Check sheet for the modelled part. Datum: model origin and axes. Units: mm. Round coordinates to 2 decimals unless told otherwise and drop trailing zeros. Write each loop counter-clockwise with the first axis right and the second up, starting at its lowest first coordinate (ties: lowest second). Pieces come first, ordered by that corner, then holes. Notation, with made-up numbers: M -8.5,39 L 8.5,39 A22 ccw 8.5,54 Z; hole C 14,82.25 d7. An arc over 180 degrees is marked long. Put each result on its own line as item: value.
```python
from build123d import *

# Parameters (mm, degrees)
F0_W = 40
F0_H = 7.5
F2_T = -1


with BuildPart() as f1:
    # F0 (on Top) → F1 (revolve)
    with BuildSketch(Plane.XY):
        with Locations((-23.359164299, 3.75)):
            Rectangle(F0_W, F0_H)
    revolve(axis=Axis((-23.359164299, 0, 0), (1, 0, 0)))

    # F2
    f2_openings = [f1.faces().sort_by_distance(p)[0] for p in [
        (-43.359164, 0, 0),
    ]]
    offset(amount=F2_T, openings=f2_openings)

    # F0 (on Top) → F3 (revolve)
    with BuildSketch(Plane.XY):
        with BuildLine():
            Line((-3.359164299, 10), (-3.359164299, 7.5))
            Line((-3.359164299, 7.5), (-3.359164299, 0))
            Line((-3.359164299, 0), (16.640835701, 0))
            add(Edge.make_bspline(
                [(13.8242446614, 5.8201136691), (15.4706541093, 3.8634896533), (16.522999446, 1.3952228585), (16.640835701, 0)],
                knots=[0.7411708943, 0.7411708943, 0.7411708943, 0.7411708943, 1, 1, 1, 1], degree=3))
            add(Edge.make_bspline(
                [(-3.359164299, 10), (-2.6756685908, 9.3742873677), (1.833779877, 8.8504755161), (9.6760817872, 9.8620826294), (13.1808157461, 6.5847767181), (13.8242446614, 5.8201136691)],
                knots=[0, 0, 0, 0, 0.2582901973, 0.6400185771, 0.7411708943, 0.7411708943, 0.7411708943, 0.7411708943], degree=3))
        make_face()
        with BuildLine():
            add(Edge.make_bspline(
                [(13.8242446614, 5.8201136691), (15.4706541093, 3.8634896533), (16.522999446, 1.3952228585), (16.640835701, 0)],
                knots=[0.7411708943, 0.7411708943, 0.7411708943, 0.7411708943, 1, 1, 1, 1], degree=3))
            Line((16.640835701, 0), (35.6210991124, 0))
            Line((35.6210991124, 0), (18.3005910367, 10))
            ThreePointArc((18.3005910367, 10), (17.4707133688, 10.4231546702), (16.640835701, 10))
            ThreePointArc((16.640835701, 10), (14.9843806263, 8.0772776447), (13.8242446614, 5.8201136691))
        make_face()
    revolve(axis=Axis((6.640835701, 0, 0), (1, 0, 0)))


solid = f1.part
```
1. Cross-section at B-B (x = 30). Enter the section's corners in (y, z), then the cut area to 3 significant figures.
Computed values:
outline: C 0,0 d6.49
area: 33.1 mm2
2. Cross-section at A-A (x = -34.5). Enter the section's corners in (y, z), then the cut area to 3 significant figures.
Computed values:
outline: C 0,0 d15; hole C 0,0 d13
area: 44.0 mm2
3. Release check for a two-part mould opening along Y. For faces 1 (the flat face through (-43.359, 6, 3)), 2 (the flat face through (-4.359, 0, 0)), 3 (the conical face through (28.764, -0.858, -3.865)) record: +Y half, -Y half, draft (parallel to the pull), parting line (faces both ways), or undercut.
Computed values:
face 1: draft
face 2: undercut
face 3: parting line
4. Scan lines: probe 1 along Z at (x, y) = (-22.5, 0); probe 2 along X at (y, z) = (0, -8.25); probe 3 along X at (y, z) = (-1.5, -8.25). Record each from-to range of solid material in increasing order.
Computed values:
probe 1: z = -7.5 to -6.5, 6.5 to 7.5
probe 2: x = -3.36 to 10.8, 15.1 to 21.33
probe 3: x = -3.36 to 10.5, 15.2 to 21.1
5. Depth check by flat-ended pin: pin 1 Ø10 at (x, y) = (-3, 2) entering from -Z; pin 2 Ø12 at (x, y) = (-22.5, 6) entering from +Z; pin 3 Ø8 at (y, z) = (-3.5, -6) entering from +X. Enter the tip coordinate at first touch or a pass-through.
Computed values:
pin 1: stops at z = -10
pin 2: stops at z = 7.5
pin 3: stops at x = 30.52
